```python
from build123d import *

# Parameters (mm, degrees)
BOSS_EXTRUDE1_DEPTH = 15
CUT_EXTRUDE1_DEPTH  = 5
SKETCH3_R           = 0.75
CUT_EXTRUDE2_DEPTH  = 30
CUT_EXTRUDE3_DEPTH  = 5


with BuildPart() as part:
    # Sketch1 → Boss-Extrude1 (new body)
    with BuildSketch(Plane(origin=(0, 0, 0), x_dir=(1, 0, 0), z_dir=(0, 1, 0))):
        Polygon((0, 0), (260, 0), (230, 30), (30, 30), align=None)
    extrude(amount=BOSS_EXTRUDE1_DEPTH)

    # Sketch2 → Cut-Extrude1 (cut)
    with BuildSketch(Plane(origin=(0, 15, 0), x_dir=(1, 0, 0), z_dir=(0, 1, 0))):
        with BuildLine():
            Line((-5, 22.5), (35, 22.5))
            ThreePointArc((35, 22.5), (42.5, 15), (35, 7.5))
            Line((35, 7.5), (-5, 7.5))
            ThreePointArc((-5, 7.5), (-12.5, 15), (-5, 22.5))
        make_face()
        with BuildLine():
            Line((265, 22.5), (225, 22.5))
            ThreePointArc((225, 22.5), (217.5, 15), (225, 7.5))
            Line((225, 7.5), (265, 7.5))
            ThreePointArc((265, 7.5), (272.5, 15), (265, 22.5))
        make_face()
    extrude(amount=-CUT_EXTRUDE1_DEPTH, mode=Mode.SUBTRACT)

    # Sketch3 → Cut-Extrude2 (cut)
    with BuildSketch(Plane.XY):
        with Locations((130, 7.5)):
            Circle(SKETCH3_R)
        with Locations((180, 7.5)):
            Circle(SKETCH3_R)
        with Locations((230, 7.5)):
            Circle(SKETCH3_R)
        with Locations((80, 7.5)):
            Circle(SKETCH3_R)
        with Locations((30, 7.5)):
            Circle(SKETCH3_R)
    extrude(amount=-CUT_EXTRUDE2_DEPTH, mode=Mode.SUBTRACT)

    # Sketch4 → Cut-Extrude3 (cut)
    with BuildSketch(Plane(origin=(0, 15, 0), x_dir=(1, 0, 0), z_dir=(0, 1, 0))):
        with BuildLine():
            Line((52.5, 25), (207.5, 25))
            ThreePointArc((207.5, 25), (211.035533906, 23.535533906), (212.5, 20))
            Line((212.5, 20), (212.5, 10))
            ThreePointArc((212.5, 10), (211.035533906, 6.464466094), (207.5, 5))
            Line((207.5, 5), (52.5, 5))
            ThreePointArc((52.5, 5), (48.964466094, 6.464466094), (47.5, 10))
            Line((47.5, 10), (47.5, 20))
            ThreePointArc((47.5, 20), (48.964466094, 23.535533906), (52.5, 25))
        make_face()
    extrude(amount=-CUT_EXTRUDE3_DEPTH, mode=Mode.SUBTRACT)


solid = part.part
```
The model under review builds one solid part; all positions refer to its coordinate system, in mm. A direction names the side the tool comes from. Round coordinates to 2 decimals unless told otherwise and drop trailing zeros. Loops run counter-clockwise (first coordinate to the right, second up) from the corner with the lowest first, then second, coordinate; pieces in that order, holes last.
Item 1: Mouldability with a two-part tool opening along Z and no side actions: class faces 5 (the face through (128, 0, -15)), 6 (the face through (128, 7, 0)), 7 (the face through (217.5, 12.54, -15.16)), 8 (the face through (15, 6, -15)) as released by +Z, released by -Z, zero draft, split by the parting line, or undercut.
Determined:
face 5: zero draft
face 6: released by +Z
face 7: undercut
face 8: released by -Z
Item 2: Take a section at B-B (x = 166). Write out the cut boundary in (y, z), then the cut area to 3 significant figures.
Determined:
outline: (0, -30) - (15, -30) - (15, -25) - (10, -25) - (10, -5) - (15, -5) - (15, 0) - (0, 0) - close
area: 350 mm2
Item 3: For faces 1 (the face through (245, 6, -15)), 2 (the face through (29, 10, -15)), 3 (the face through (129, 13, -25)), 4 (the face through (239, 13, -7.5)), list the 3-axis set-ups (+Z, -Z, +X, -X, +Y, -Y) from which the entire face can be reached by the end or side of a thin tool; tool diameter is ignored.
Determined:
face 1: -Z, +X, +Y, -Y
face 2: -X, +Y
face 3: +Y
face 4: +X, +Y
Item 4: Clearance check with flat-ended pins moving along their axes: pin 1 Ø1.2 at (x, y) = (130, 7.5) entering from -Z; pin 2 Ø1.5 at (x, y) = (236, 12) entering from -Z; pin 3 Ø1 at (y, z) = (11.5, -9) entering from +X; pin 4 Ø4.5 at (x, z) = (21.5, -12) entering from +Y. State where each tip first meets the part, or that it passes through.
Determined:
pin 1: passes through
pin 2: stops at z = -24.75
pin 3: stops at x = 221.26
pin 4: stops at y = 10
Item 5: Take a section at A-A (y = 12.5). Write out the cut boundary in (x, z).
Determined:
outline: (0, 0) - (7.5, -7.5) - (35, -7.5) arc R7.5 cw to (35, -22.5) - (22.5, -22.5) - (30, -30) - (230, -30) - (237.5, -22.5) - (225, -22.5) arc R7.5 cw to (225, -7.5) - (252.5, -7.5) - (260, 0) - close; hole (47.5, -20) arc R5 ccw to (52.5, -25) - (207.5, -25) arc R5 ccw to (212.5, -20) - (212.5, -10) arc R5 ccw to (207.5, -5) - (52.5, -5) arc R5 ccw to (47.5, -10) - close
Item 6: For line 1 (Z direction, x = 71, y = 12.5); line 2 (Y direction, x = 130, z = -8); line 3 (Y direction, x = 30, z = -23.25), list the stretches that pass through material, from the lowest coordinate up.
Determined:
line 1: z = -30 to -25, -5 to 0
line 2: y = 0 to 6.75, 8.25 to 10
line 3: y = 0 to 6.75, 8.25 to 15
